```python
from build123d import *

# Parameters (mm, degrees)
SKETCH_1_W          = 10
SKETCH_1_H          = 3
EXTRUDE_1_DEPTH     = 10
SKETCH_2_R          = 3.2
CUT_EXTRUDE_1_DEPTH = 8
SKETCH_3_R          = 1.75
CUT_EXTRUDE_2_DEPTH = 4
FILLET_1_R          = 3
FILLET_2_R          = 1


with BuildPart() as part:
    # ｽｹｯﾁ1 → ﾎﾞｽ - 押し出し1 (new body)
    with BuildSketch(Plane.XY):
        Polygon((5, 10), (0, 10), (0, -5), (5, -5), (5, 7), align=None)
        with Locations((10, 8.5)):
            Rectangle(SKETCH_1_W, SKETCH_1_H)
        Polygon((0, -5), (0, 10), (-5, 10), (-5, 7), (-5, -5), align=None)
        with Locations((-10, 8.5)):
            Rectangle(SKETCH_1_W, SKETCH_1_H)
    extrude(amount=EXTRUDE_1_DEPTH)

    # ｽｹｯﾁ2 → ｶｯﾄ - 押し出し1 (cut)
    with BuildSketch(Plane(origin=(0, 0, 0), x_dir=(-1, 0, 0), z_dir=(0, 0, -1))):
        Circle(SKETCH_2_R)
    extrude(amount=-CUT_EXTRUDE_1_DEPTH, mode=Mode.SUBTRACT)

    # ｽｹｯﾁ3 → ｶｯﾄ - 押し出し2 (cut, through all)
    with BuildSketch(Plane.XZ.offset(-7)):
        with Locations((-11.5, 5)):
            Circle(SKETCH_3_R)
        with Locations((11.5, 5)):
            Circle(SKETCH_3_R)
    extrude(amount=-CUT_EXTRUDE_2_DEPTH, mode=Mode.SUBTRACT)

    # ﾌｨﾚｯﾄ1
    fillet_1_edges = [part.edges().sort_by_distance(p)[0] for p in [
        (5, -5, 5),
        (-5, -5, 5),
        (-5, 7, 5),
        (5, 7, 5),
    ]]
    fillet(fillet_1_edges, radius=FILLET_1_R)

    # ﾌｨﾚｯﾄ2
    fillet_2_edges = [part.edges().sort_by_distance(p)[0] for p in [
        (-15, 8.5, 0),
        (15, 8.5, 0),
        (15, 8.5, 10),
        (-15, 7, 5),
        (15, 7, 5),
        (-15, 8.5, 10),
        (-5, 1, 0),
        (-5, 1, 10),
        (-11.5, 7, 0),
        (-11.5, 7, 10),
        (11.5, 7, 0),
        (11.5, 7, 10),
        (5, 1, 0),
        (5, 1, 10),
        (0, -5, 0),
        (0, -5, 10),
        (4.121320344, -4.121320344, 0),
        (-4.121320344, -4.121320344, 0),
        (4.121320344, -4.121320344, 10),
        (-4.121320344, -4.121320344, 10),
        (-5.878679656, 6.121320344, 0),
        (-5.878679656, 6.121320344, 10),
        (5.878679656, 6.121320344, 0),
        (5.878679656, 6.121320344, 10),
    ]]
    fillet(fillet_2_edges, radius=FILLET_2_R)


solid = part.part
```
Check sheet for the modelled part. Datum: model origin and axes. Units: mm. A direction names the side the tool comes from. Round coordinates to 2 decimals unless told otherwise and drop trailing zeros. Order: outer loops, then holes, each group sorted by start corner. A loop starts at its lowest first (then second) coordinate and runs counter-clockwise, first axis right, second up. Notation, with made-up numbers: (68.25, 56) -> (99.25, 56) arc R21 cw to (99.25, 67) -> close; hole circle Ø6 at (22, -15). An arc over 180 degrees is marked (long way). Use CSV: the item, a comma, the result in double quotes.
(1) Draft check along X on faces 6 (the face through (4.699, 1.042, 0.285)), 7 (the face through (0, 5, 10)), 8 (the face through (-10.69, 8.48, 3.45)), 9 (the face through (12.31, 8.48, 3.45)). Enter one of: pulls with the +X half, pulls with the -X half, needs draft (parallel to the pull), parting line crosses it, or undercut.
Worked out:
face 6,"pulls with the +X half"
face 7,"needs draft"
face 8,"undercut"
face 9,"undercut"
(2) Cross-section at A-A (z = 5). Record the boundary of the cut face in (x, y), and give its area (3 significant figures).
Worked out:
outline,"(-15, 8) arc R1 ccw to (-14, 7) -> (-13.25, 7) -> (-13.25, 10) -> (-15, 10) -> close; (-9.75, 7) -> (-8, 7) arc R3 cw to (-5, 4) -> (-5, -2) arc R3 ccw to (-2, -5) -> (2, -5) arc R3 ccw to (5, -2) -> (5, 4) arc R3 cw to (8, 7) -> (9.75, 7) -> (9.75, 10) -> (-9.75, 10) -> close; (13.25, 7) -> (14, 7) arc R1 ccw to (15, 8) -> (15, 10) -> (13.25, 10) -> close; hole circle Ø6.4 at (0, 0)"
area,"156 mm²"
(3) Material ranges on line 1 along Y through (x, z) = (0, 2.5); line 2 along Z through (x, y) = (-11.5, 9.1); line 3 along X through (y, z) = (2, 9), recorded low to high. Write a range as from..to.
Worked out:
line 1,"-5..-3.2, 3.2..10"
line 2,"0..3.25, 6.75..10"
line 3,"-5..5"
(4) Depth check by flat-ended pin: pin 1 (4.5 mm diameter, centred on x = 11.5, z = 5, fed in from -Y); pin 2 (1 mm diameter, centred on y = -1, z = 4.5, fed in from +X); pin 3 (5 mm diameter, centred on y = 7.5, z = 3, fed in from +X); pin 4 (3 mm diameter, centred on x = 0, y = -1.5, fed in from -Z). Enter the tip coordinate at first touch or a pass-through.
Worked out:
pin 1,"y = 7"
pin 2,"x = 5"
pin 3,"x = 15"
pin 4,"z = 8"
(5) Cross-section at D-D (y = 0). Record the boundary of the cut face in (x, z).
Worked out:
outline,"(-5, 1) arc R1 ccw to (-4, 0) -> (-3.2, 0) -> (-3.2, 8) -> (3.2, 8) -> (3.2, 0) -> (4, 0) arc R1 ccw to (5, 1) -> (5, 9) arc R1 ccw to (4, 10) -> (-4, 10) arc R1 ccw to (-5, 9) -> close"
(6) Tool access check on faces 1 (the face through (9.6, 7, 4.9)), 2 (the face through (-5, 1, 5)), 3 (the face through (2.539, -1.947, 3.944)), 4 (the face through (-10.958, 7.301, 9.715)), 5 (the face through (-10.958, 7.301, 0.285)). Record the directions out of +Z, -Z, +X, -X, +Y, -Y that give a thin tool (end or side, any length) a straight path to the whole face; none if there is none.
Worked out:
face 1,"+Z, -Z, +X, -Y"
face 2,"+Z, -Z, -X, -Y"
face 3,"-Z"
face 4,"+Z, -X, -Y"
face 5,"-Z, -X, -Y"
(7) Cross-section at C-C (z = 2.5). Record the boundary of the cut face in (x, y).
Worked out:
outline,"(-15, 8) arc R1 ccw to (-14, 7) -> (-8, 7) arc R3 cw to (-5, 4) -> (-5, -2) arc R3 ccw to (-2, -5) -> (2, -5) arc R3 ccw to (5, -2) -> (5, 4) arc R3 cw to (8, 7) -> (14, 7) arc R1 ccw to (15, 8) -> (15, 10) -> (-15, 10) -> close; hole circle Ø6.4 at (0, 0)"
(8) Cross-section at B-B (x = -11.5). Record the boundary of the cut face in (y, z).
Worked out:
outline,"(7, 1) arc R1 ccw to (8, 0) -> (10, 0) -> (10, 3.25) -> (7, 3.25) -> close; (7, 6.75) -> (10, 6.75) -> (10, 10) -> (8, 10) arc R1 ccw to (7, 9) -> close"
